```python
from build123d import *

# Parameters (mm, degrees)
SKETCH1_W           = 44.8
SKETCH1_H           = 19.8
BOSS_EXTRUDE1_DEPTH = 5
SKETCH2_R           = 1.1
CUT_EXTRUDE1_DEPTH  = 13
SKETCH3_R           = 1.5
CUT_EXTRUDE2_DEPTH  = 10
FILLET1_R           = 30
SKETCH4_W           = 13
SKETCH4_H           = 10
CUT_EXTRUDE3_DEPTH  = 10
BOSS_EXTRUDE2_START = -5
SKETCH5_R           = 2
SKETCH5_R_2         = 1.5
BOSS_EXTRUDE2_DEPTH = 5
FILLET2_R           = 0.5


with BuildPart() as part:
    # Sketch1 → Boss-Extrude1 (new body)
    with BuildSketch(Plane.XY):
        with Locations((0, 19.08)):
            Rectangle(SKETCH1_W, SKETCH1_H)
    extrude(amount=BOSS_EXTRUDE1_DEPTH)

    # Sketch2 → Cut-Extrude1 (cut)
    with BuildSketch(Plane.XY.offset(5)):
        with Locations((-20, 25)):
            Circle(SKETCH2_R)
        with Locations((-20, 13)):
            Circle(SKETCH2_R)
        with Locations((20, 25)):
            Circle(SKETCH2_R)
        with Locations((20, 13)):
            Circle(SKETCH2_R)
    extrude(amount=-CUT_EXTRUDE1_DEPTH, mode=Mode.SUBTRACT)

    # Sketch3 → Cut-Extrude2 (cut)
    with BuildSketch(Plane.XY.offset(5)):
        with Locations((-8.5, 19)):
            Circle(SKETCH3_R)
        with Locations((8.5, 19)):
            Circle(SKETCH3_R)
    extrude(amount=-CUT_EXTRUDE2_DEPTH, mode=Mode.SUBTRACT)

    # Fillet1
    # the kernel refuses this fillet: 30 mm, written as the material it takes off along each edge
    with BuildSketch(Plane(origin=(22.4, -32.277809879, 5), x_dir=(0, 0, -1), z_dir=(0, 1, 0)), Plane(origin=(-22.4, 70.437809879, 5), x_dir=(0, 0, -1), z_dir=(0, -1, 0))) as fillet1_piece_1:
        with BuildLine():
            CenterArc((30, 16.583123952), FILLET1_R, 180, 33.557309762)
            Line((0, 16.583123952), (-0.6, 16.583123952))
            Line((-0.6, 16.583123952), (-0.6, 0))
            Line((-0.6, 0), (0, -0.6))
            ThreePointArc((0, -0.6), (2.5, -0.6), (4.5, -0.331662479))
            Line((4.5, -0.331662479), (5, 0))
        make_face()
    extrude(amount=102.715619759, mode=Mode.SUBTRACT)

    # Sketch4 → Cut-Extrude3 (cut)
    with BuildSketch(Plane.XY.offset(5)):
        with Locations((0, 19)):
            Rectangle(SKETCH4_W, SKETCH4_H)
    extrude(amount=-CUT_EXTRUDE3_DEPTH, mode=Mode.SUBTRACT)

    # Sketch5 → Boss-Extrude2 (add)
    # profile 1 of 6: a face of its own
    with BuildSketch(Plane(origin=(0, 0, 0), x_dir=(-1, 0, 0), z_dir=(0, 0, -1)).offset(BOSS_EXTRUDE2_START)):
        with Locations((-8.5, 19)):
            Circle(SKETCH5_R)
        with Locations((-8.5, 19)):
            Circle(SKETCH5_R_2, mode=Mode.SUBTRACT)
    # profile 2 of 6: a face of its own
    with BuildSketch(Plane(origin=(0, 0, 0), x_dir=(-1, 0, 0), z_dir=(0, 0, -1)).offset(BOSS_EXTRUDE2_START)):
        with BuildLine():
            Line((-6.5, 21), (-8.5, 21))
            ThreePointArc((-8.5, 21), (-7.085786438, 20.414213562), (-6.5, 19))
            Line((-6.5, 19), (-6.5, 21))
        make_face()
    # profile 3 of 6: a face of its own
    with BuildSketch(Plane(origin=(0, 0, 0), x_dir=(-1, 0, 0), z_dir=(0, 0, -1)).offset(BOSS_EXTRUDE2_START)):
        with BuildLine():
            Line((-6.5, 17), (-6.5, 19))
            ThreePointArc((-6.5, 19), (-7.085786438, 17.585786438), (-8.5, 17))
            Line((-8.5, 17), (-6.5, 17))
        make_face()
    # profile 4 of 6: a face of its own
    with BuildSketch(Plane(origin=(0, 0, 0), x_dir=(-1, 0, 0), z_dir=(0, 0, -1)).offset(BOSS_EXTRUDE2_START)):
        with Locations((8.5, 19)):
            Circle(SKETCH5_R)
        with Locations((8.5, 19)):
            Circle(SKETCH5_R_2, mode=Mode.SUBTRACT)
    # profile 5 of 6: a face of its own
    with BuildSketch(Plane(origin=(0, 0, 0), x_dir=(-1, 0, 0), z_dir=(0, 0, -1)).offset(BOSS_EXTRUDE2_START)):
        with BuildLine():
            ThreePointArc((8.5, 17), (7.08578644, 17.585786436), (6.5, 18.999999994))
            Line((6.5, 18.999999994), (6.5, 17))
            Line((6.5, 17), (8.5, 17))
        make_face()
    # profile 6 of 6: a face of its own
    with BuildSketch(Plane(origin=(0, 0, 0), x_dir=(-1, 0, 0), z_dir=(0, 0, -1)).offset(BOSS_EXTRUDE2_START)):
        with BuildLine():
            ThreePointArc((6.5, 18.999999994), (7.085786436, 20.41421356), (8.5, 21))
            Line((8.5, 21), (6.5, 21))
            Line((6.5, 21), (6.5, 18.999999994))
        make_face()
    extrude(amount=BOSS_EXTRUDE2_DEPTH)

    # Fillet2
    fillet2_edges = [part.edges().sort_by_distance(p)[0] for p in [
        (-6.5, 14, 2.496110676),
        (-6.5, 24, 2.496110676),
        (6.5, 24, 2.496110676),
        (6.5, 14, 2.496110676),
    ]]
    fillet(fillet2_edges, radius=FILLET2_R)


solid = part.part
```
The model under review builds one solid part; all positions refer to its coordinate system, in mm. A direction names the side the tool comes from. Coordinates: 2 decimals unless noted, no trailing zeros. Order: outer loops, then holes, each group sorted by start corner. A loop starts at its lowest first (then second) coordinate and runs counter-clockwise, first axis right, second up. Notation, with made-up numbers: (48, 79) -> (71, 79) arc R30 cw to (71, 111) -> close; hole circle Ø1 at (-34.5, -18). An arc over 180 degrees is marked (long way). Answer in a Markdown table with one row per item. Add a question column.
Item 1: We need section A-A on x = -2. Write out the cut boundary in (y, z).
Item 2: Mouldability with a two-part tool opening along X and no side actions: class faces 4 (the flat face through (0, 14, 3)), 5 (the flat face through (0, 27, 5)), 6 (the cylindrical face through (-10.5, 19, 4.8)) as +X half, -X half, draft (parallel to the pull), parting line (faces both ways), or undercut.
Item 3: We need section D-D on y = 25. Write out the cut boundary in (x, z), plus the area to 3 significant figures.
Item 4: Machinability: for faces 1 (the flat face through (-6.5, 19, 3)), 2 (the cylindrical face through (10.5, 19, 4.8)), 3 (the flat face through (7, 18, 5)), which of the approach directions +Z, -Z, +X, -X, +Y, -Y give a long, thin tool a straight path to every point of the face, cutting with its end or side? Answer none if there is none.
Item 5: To check wall thickness, follow probe 1 along X at (y, z) = (19, 4.85); probe 2 along Y at (x, z) = (8.5, 1.5); probe 3 along X at (y, z) = (25, 0.7). State the ranges of each line that lie inside material, in increasing order.
Item 6: Clearance check with flat-ended pins moving along their axes: pin 1 (1.5 mm diameter, centred on y = 23, z = 3.5, fed in from -X); pin 2 (3.5 mm diameter, centred on x = 8.5, y = 19, fed in from +Z); pin 3 (2.5 mm diameter, centred on y = 20, z = 2.5, fed in from +X); pin 4 (2 mm diameter, centred on x = -20, y = 13, fed in from +Z). State where each tip first meets the part, or that it passes through.
Item 7: We need section C-C on z = 2.4. Write out the cut boundary in (x, y), plus the area to 3 significant figures.
Item 8: We need section B-B on y = 19. Write out the cut boundary in (x, z), plus the area to 3 significant figures.
Final values:
| question | item | result |
|---|---|---|
| 1 | outline | (9.18, 0) -> (14, 0) -> (14, 5) -> (9.18, 5) -> close; (24, 0) -> (28.98, 0) -> (28.98, 5) -> (24, 5) -> close |
| 2 | face 4 | undercut |
| 2 | face 5 | draft |
| 2 | face 6 | -X half |
| 3 | outline | (-22.4, 0) -> (-21.1, 0) -> (-21.1, 0.82) arc R30 ccw to start; (-18.9, 0) -> (18.9, 0) -> (18.9, 2) arc R30 ccw to (5.82, 5) -> (-5.82, 5) arc R30 ccw to (-18.9, 2) -> close; (21.1, 0) -> (22.4, 0) arc R30 ccw to (21.1, 0.82) -> close |
| 3 | area | 164 mm2 |
| 4 | face 1 | +Z, -Z |
| 4 | face 2 | +Z, +X |
| 4 | face 3 | +Z, +X, -X, +Y, -Y |
| 5 | probe 1 | x = -10.5 to -10, -7 to -6.5, 6.5 to 7, 10 to 10.5 |
| 5 | probe 2 | y = 9.18 to 17.5, 20.5 to 28.98 |
| 5 | probe 3 | x = -21.29 to -21.1, -18.9 to 18.9, 21.1 to 21.29 |
| 6 | pin 1 | stops at x = -17.22 |
| 6 | pin 2 | stops at z = 5 |
| 6 | pin 3 | stops at x = 20.34 |
| 6 | pin 4 | passes through |
| 7 | outline | (-18.03, 9.18) -> (18.03, 9.18) -> (18.03, 28.98) -> (-18.03, 28.98) -> close; hole circle Ø3 at (-8.5, 19); hole (-6.5, 14.5) arc R0.5 ccw to (-6, 14) -> (6, 14) arc R0.5 ccw to (6.5, 14.5) -> (6.5, 23.5) arc R0.5 ccw to (6, 24) -> (-6, 24) arc R0.5 ccw to (-6.5, 23.5) -> close; hole circle Ø3 at (8.5, 19) |
| 7 | area | 570 mm2 |
| 8 | outline | (-22.4, 0) -> (-10, 0) -> (-10, 5) -> (-10.5, 5) -> (-10.5, 4.63) arc R30 ccw to start; (-7, 0) -> (-6.5, 0) -> (-6.5, 5) -> (-7, 5) -> close; (6.5, 0) -> (7, 0) -> (7, 5) -> (6.5, 5) -> close; (10, 0) -> (22.4, 0) arc R30 ccw to (10.5, 4.63) -> (10.5, 5) -> (10, 5) -> close |
| 8 | area | 76.9 mm2 |
